Geometry check sheet. Reference: the model listing, model coordinates, mm. A direction names the side the tool comes from. Round coordinates to 2 decimals unless told otherwise and drop trailing zeros. Order: outer loops, then holes, each group sorted by start corner. A loop starts at its lowest first (then second) coordinate and runs counter-clockwise, first axis right, second up. Notation, with made-up numbers: (33.5, -4) - (64.5, -4) arc R31 cw to (64.5, 32) - close; hole circle Ø1 at (-5.5, 0.25). An arc over 180 degrees is marked (long way). Use a Markdown table: item, result. Add a question column.
(1) Section check C-C on y = -10.5. Record the boundary of the cut face in (x, z).
(2) Section check A-A on z = 19. Record the boundary of the cut face in (x, y), then the cut area to 3 significant figures.
(3) Thickness scan on line 1 along Z through (x, y) = (15.5, 27); line 2 along Y through (x, z) = (5, 57); line 3 along X through (y, z) = (-6, 11). Record the ranges inside material, lowest first. Write a range as [from, to].
(4) Gauge pin test, flat ends, axial feed: P1, Ø6.5, axis at x = -10, z = 64.14, coming from the +Y side; P2, Ø2, axis at x = 36.82, y = 28.2, coming from the +Z side; P3, Ø4, axis at x = -17, y = 12.5, coming from the -Z side; P4, Ø21, axis at x = 9, z = 62, coming from the -Y side. Record the tip position at first contact, or that the pin passes through.
(5) Section check B-B on y = 0. Record the boundary of the cut face in (x, z), then the cut area to 3 significant figures.
(6) Mould release check, pull along Z, two halves, no side actions. Record for faces 5 (the face through (-10.26, 4.528, 62.157)), 6 (the face through (1, 1, 0)), 7 (the face through (36.03, 35.81, 3.7)): released by +Z, released by -Z, zero draft, split by the parting line, or undercut.
(7) Access from +Z, -Z, +X, -X, +Y, -Y to the whole of each face (thin tool, end or side, straight path). Record for faces 1 (the face through (10.427, -25.391, 3.698)), 2 (the face through (-25, 0, 4)), 3 (the face through (18.865, 32.708, 3.698)), 4 (the face through (25.391, 10.427, 3.698)).
```python
from build123d import *

# Parameters (mm, degrees)
SKETCH8_R           = 1.266
BOSS_EXTRUDE3_DEPTH = 7.5
BOSS_EXTRUDE4_DEPTH = 20
SKETCH10_R          = 2
CUT_EXTRUDE3_DEPTH  = 13


with BuildPart() as part:
    # Sketch8 → Boss-Extrude3 (new body)
    with BuildSketch(Plane.XY):
        with BuildLine():
            Line((-26.464466094, 12.621101614), (-39.129662609, 25.286298129))
            ThreePointArc((-39.129662609, 25.286298129), (-40.587272547, 28.560079176), (-39.479950614, 31.968320248))
            ThreePointArc((-39.479950614, 31.968320248), (-35.753947361, 36.087328082), (-31.600536501, 39.774943028))
            ThreePointArc((-31.600536501, 39.774943028), (-28.205326911, 40.851961857), (-24.954713569, 39.395620337))
            Line((-24.954713569, 39.395620337), (-12.023559327, 26.464466094))
            ThreePointArc((-12.023559327, 26.464466094), (-10.401442583, 25.380602337), (-8.488025421, 25))
            Line((-8.488025421, 25), (9.085567708, 25))
            ThreePointArc((9.085567708, 25), (10.99898487, 25.380602337), (12.621101614, 26.464466094))
            Line((12.621101614, 26.464466094), (25.286298129, 39.129662609))
            ThreePointArc((25.286298129, 39.129662609), (28.560079176, 40.587272547), (31.968320248, 39.479950614))
            ThreePointArc((31.968320248, 39.479950614), (36.087328082, 35.753947361), (39.774943028, 31.600536501))
            ThreePointArc((39.774943028, 31.600536501), (40.851961857, 28.205326911), (39.395620337, 24.954713569))
            Line((39.395620337, 24.954713569), (26.464466094, 12.023559327))
            ThreePointArc((26.464466094, 12.023559327), (25.380602337, 10.401442583), (25, 8.488025421))
            Line((25, 8.488025421), (25, -9.085567708))
            ThreePointArc((25, -9.085567708), (25.380602337, -10.99898487), (26.464466094, -12.621101614))
            Line((26.464466094, -12.621101614), (39.129662609, -25.286298129))
            ThreePointArc((39.129662609, -25.286298129), (40.587272547, -28.560079176), (39.479950614, -31.968320248))
            ThreePointArc((39.479950614, -31.968320248), (35.753947361, -36.087328082), (31.600536501, -39.774943028))
            ThreePointArc((31.600536501, -39.774943028), (28.205326911, -40.851961857), (24.954713569, -39.395620337))
            Line((24.954713569, -39.395620337), (12.023559327, -26.464466094))
            ThreePointArc((12.023559327, -26.464466094), (10.401442583, -25.380602337), (8.488025421, -25))
            Line((8.488025421, -25), (-9.085567708, -25))
            ThreePointArc((-9.085567708, -25), (-10.99898487, -25.380602337), (-12.621101614, -26.464466094))
            Line((-12.621101614, -26.464466094), (-25.286298129, -39.129662609))
            ThreePointArc((-25.286298129, -39.129662609), (-28.560079176, -40.587272547), (-31.968320248, -39.479950614))
            ThreePointArc((-31.968320248, -39.479950614), (-36.087328082, -35.753947361), (-39.774943028, -31.600536501))
            ThreePointArc((-39.774943028, -31.600536501), (-40.851961857, -28.205326911), (-39.395620337, -24.954713569))
            Line((-39.395620337, -24.954713569), (-26.464466094, -12.023559327))
            ThreePointArc((-26.464466094, -12.023559327), (-25.380602337, -10.401442583), (-25, -8.488025421))
            Line((-25, -8.488025421), (-25, 9.085567708))
            ThreePointArc((-25, 9.085567708), (-25.380602337, 10.99898487), (-26.464466094, 12.621101614))
        make_face()
        with Locations((-28.19800422, -36.819050096)):
            Circle(SKETCH8_R, mode=Mode.SUBTRACT)
        with Locations((-36.819050096, -28.19800422)):
            Circle(SKETCH8_R, mode=Mode.SUBTRACT)
        with Locations((-36.819050096, 28.19800422)):
            Circle(SKETCH8_R, mode=Mode.SUBTRACT)
        with Locations((-28.19800422, 36.819050096)):
            Circle(SKETCH8_R, mode=Mode.SUBTRACT)
        with Locations((28.19800422, 36.819050096)):
            Circle(SKETCH8_R, mode=Mode.SUBTRACT)
        with Locations((36.819050096, 28.19800422)):
            Circle(SKETCH8_R, mode=Mode.SUBTRACT)
        with Locations((36.819050096, -28.19800422)):
            Circle(SKETCH8_R, mode=Mode.SUBTRACT)
        with Locations((28.19800422, -36.819050096)):
            Circle(SKETCH8_R, mode=Mode.SUBTRACT)
    extrude(amount=BOSS_EXTRUDE3_DEPTH)

    # Sketch9 → Boss-Extrude4 (add, symmetric)
    with BuildSketch(Plane(origin=(0, 0, 0), x_dir=(0, 0, -1), z_dir=(1, 0, 0))):
        with BuildLine():
            Line((-7.5, -25), (-7.5, 25))
            Line((-7.5, 25), (-32.5, 25))
            ThreePointArc((-32.5, 25), (-47.706906326, 19.843134833), (-56.640215409, 6.5))
            Line((-56.640215409, 6.5), (-71.640215409, 6.5))
            Line((-71.640215409, 6.5), (-71.640215409, 2.5))
            Line((-71.640215409, 2.5), (-52.343134833, 2.5))
            ThreePointArc((-52.343134833, 2.5), (-12.5, 0), (-52.343134833, -2.5))
            Line((-52.343134833, -2.5), (-71.640215409, -2.5))
            Line((-71.640215409, -2.5), (-71.640215409, -6.5))
            Line((-71.640215409, -6.5), (-56.640215409, -6.5))
            ThreePointArc((-56.640215409, -6.5), (-47.706906326, -19.843134833), (-32.5, -25))
            Line((-32.5, -25), (-7.5, -25))
        make_face()
    extrude(amount=BOSS_EXTRUDE4_DEPTH, both=True)

    # Sketch10 → Cut-Extrude3 (cut)
    with BuildSketch(Plane(origin=(0, 6.5, 0), x_dir=(1, 0, 0), z_dir=(0, 1, 0))):
        with Locations((-10, -64.140215409)):
            Circle(SKETCH10_R)
        with Locations((10, -64.140215409)):
            Circle(SKETCH10_R)
    extrude(amount=-CUT_EXTRUDE3_DEPTH, mode=Mode.SUBTRACT)


solid = part.part
```
Check sheet entries:
| question | item | result |
|---|---|---|
| 1 | outline | (-25.42, 0) - (25.2, 0) - (25.2, 7.5) - (20, 7.5) - (20, 15.48) - (-20, 15.48) - (-20, 7.5) - (-25.42, 7.5) - close; (-20, 49.52) - (20, 49.52) - (20, 55.19) - (-20, 55.19) - close |
| 2 | outline | (-20, -25) - (20, -25) - (20, -14.76) - (-20, -14.76) - close; (-20, 14.76) - (20, 14.76) - (20, 25) - (-20, 25) - close |
| 2 | area | 819 mm2 |
| 3 | line 1 | z = [0, 7.5] |
| 3 | line 2 | y = [-6.5, -2.5], [2.5, 6.5] |
| 3 | line 3 | x = [-20, 20] |
| 4 | P1 | stops at y = 6.5 |
| 4 | P2 | passes through |
| 4 | P3 | stops at z = 0 |
| 4 | P4 | stops at y = -16.25 |
| 5 | outline | (-25, 0) - (25, 0) - (25, 7.5) - (20, 7.5) - (20, 12.5) - (-20, 12.5) - (-20, 7.5) - (-25, 7.5) - close |
| 5 | area | 575 mm2 |
| 6 | face 5 | undercut |
| 6 | face 6 | released by -Z |
| 6 | face 7 | zero draft |
| 7 | face 1 | +Z, -Z, -Y |
| 7 | face 2 | +Z, -Z, -X |
| 7 | face 3 | +Z, -Z, +Y |
| 7 | face 4 | +Z, -Z, +X |
